Could you check a few things on this model? Use its own coordinates, in mm. Face numbers are marked on the shaded views. A direction names the side the tool comes from. Give positions to 0.01 mm unless a question says otherwise; leave off trailing zeros. Write each loop counter-clockwise with the first axis right and the second up, starting at its lowest first coordinate (ties: lowest second). Pieces come first, ordered by that corner, then holes. Notation, with made-up numbers: M 12.5,30 L 71.5,30 A21 ccw 71.5,36 Z; hole C 64,5.25 d7. An arc over 180 degrees is marked long. Answer as CSV lines item,"result". Start each with the question number.
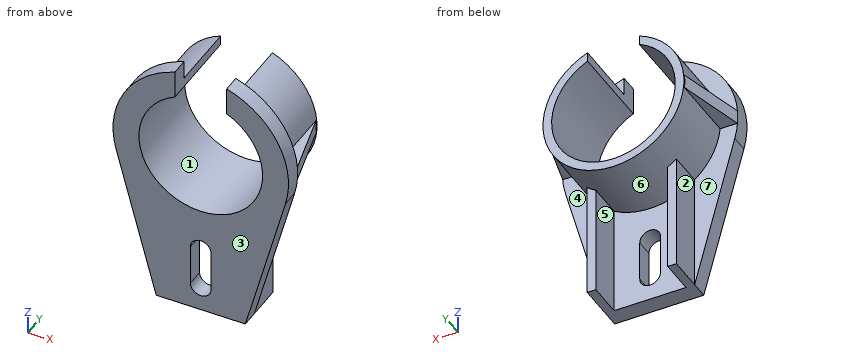
from build123d import *

# Parameters (mm, degrees)
SKETCH8_R           = 11.3665
BOSS_EXTRUDE3_DEPTH = 3.175
SKETCH9_R           = 12.954
SKETCH9_R_2         = 11.3665
BOSS_EXTRUDE4_DEPTH = 12.7
RIB12_REACH         = 40.783
SKETCH13_WALL_W     = 92.662520058
SKETCH13_WALL_H     = 2.54
CUT_EXTRUDE1_DEPTH  = 52.861115163
RIB1_START          = -47.625
RIB1_OUTLINE_W      = 1.5875
RIB1_OUTLINE_H      = 6.35
RIB1_DEPTH          = 21.4607898
SKETCH16_W          = 9.525
SKETCH16_H          = 15.588386278
CUT_EXTRUDE3_DEPTH  = 53.72855859


# Read off the part's stored shape, not the designer's step: Rib1
with BuildPart() as part:
    # Sketch8 → Boss-Extrude3 (new body)
    with BuildSketch(Plane(origin=(0, 0, 0), x_dir=(1, 0, 0), z_dir=(0, 1, 0))):
        with BuildLine():
            Line((-8.1915, 47.625), (8.1915, 47.625))
            Line((8.1915, 47.625), (15.569804863, 20.339203977))
            ThreePointArc((15.569804863, 20.339203977), (0, 0), (-15.569804863, 20.339203977))
            Line((-15.569804863, 20.339203977), (-8.1915, 47.625))
        make_face()
        with Locations(Location((0, 16.129, 0), (0, 0, 270))):
            Circle(SKETCH8_R, mode=Mode.SUBTRACT)
    extrude(amount=BOSS_EXTRUDE3_DEPTH)

    # Sketch9 → Boss-Extrude4 (add)
    with BuildSketch(Plane(origin=(0, 3.175, 0), x_dir=(1, 0, 0), z_dir=(0, 1, 0))):
        with Locations(Location((0, 16.129, 0), (0, 0, 270))):
            Circle(SKETCH9_R)
        with Locations(Location((0, 16.129, 0), (0, 0, 270))):
            Circle(SKETCH9_R_2, mode=Mode.SUBTRACT)
    extrude(amount=BOSS_EXTRUDE4_DEPTH)

    # Sketch13 wall → Rib12 (add, up to next)
    with BuildSketch(Plane(origin=(-14.453521799, 9.525, -16.129), x_dir=(-0.243924343996, -0.969794263958, 0), z_dir=(0.969794263958, -0.243924343996, 0)), mode=Mode.PRIVATE) as rib12_sk1:
        Rectangle(SKETCH13_WALL_W, SKETCH13_WALL_H)
    rib12_tool1 = extrude(rib12_sk1.sketch, amount=RIB12_REACH, mode=Mode.PRIVATE) - part.part
    rib12 = rib12_tool1.solids().sort_by_distance((-14.453521799, 9.525, -16.129))[0]
    add(rib12)

    # Mirror2: Rib12 across plane
    add(rib12.mirror(Plane(origin=(0, 0, 0), x_dir=(0, 0, 1), z_dir=(1, 0, 0))))

    # Sketch11 → Cut-Extrude1 (cut, through all)
    with BuildSketch(Plane(origin=(0, 3.175, 0), x_dir=(1, 0, 0), z_dir=(0, 1, 0))):
        with BuildLine():
            Line((1.89865, 42.8625), (1.89865, 35.433))
            ThreePointArc((1.89865, 35.433), (0, 33.53435), (-1.89865, 35.433))
            Line((-1.89865, 35.433), (-1.89865, 42.8625))
            ThreePointArc((-1.89865, 42.8625), (0, 44.76115), (1.89865, 42.8625))
        make_face()
    extrude(amount=-CUT_EXTRUDE1_DEPTH, mode=Mode.SUBTRACT)

    # Rib1 outline → Rib1 (add)
    with BuildSketch(Plane.XY.offset(RIB1_START)):
        with Locations((-7.39775, 6.35)):
            Rectangle(RIB1_OUTLINE_W, RIB1_OUTLINE_H)
    rib1 = extrude(amount=RIB1_DEPTH)

    # Mirror1: Rib1 across plane
    add(rib1.mirror(Plane(origin=(0, 0, 0), x_dir=(0, 0, 1), z_dir=(1, 0, 0))))

    # Sketch16 → Cut-Extrude3 (cut, through all)
    with BuildSketch(Plane(origin=(0, 0, 0), x_dir=(1, 0, 0), z_dir=(0, 1, 0))):
        Rectangle(SKETCH16_W, SKETCH16_H)
    extrude(amount=CUT_EXTRUDE3_DEPTH, mode=Mode.SUBTRACT)


solid = part.part
1. Imagine slicing it at C-C, the plane z = -6.5. Please give me the cut outline in (x, y) (3 decimals), plus the area to 4 significant figures.
2. On a 3-axis mill with a long thin cutter (end or side, diameter ignored), from which of +Z, -Z, +X, -X, +Y, -Y can I reach the whole of each face in a straight line? I mean the marked faces 4, 5, 6 and 7. Say none if no direction works.
3. Imagine slicing it at D-D, the plane x = -6. Please give me the cut outline in (y, z) (3 decimals).
4. Will these pins go through, and if not, where does the flat tip stop? P1, Ø14.5, axis at x = -0.5, z = -34, coming from the +Y side (3 decimals); P2, Ø4, axis at y = 8.5, z = -4.5, coming from the +X side; P3, Ø0.8, axis at x = 7.5, z = -36, coming from the +Y side (3 decimals); P4, Ø1.6, axis at y = 2, z = -39, coming from the -X side.
5. Imagine slicing it at A-A, the plane x = 0. Please give me the cut outline in (y, z) (1 decimal), plus the area to 3 significant figures.
6. Thinking about a two-plate mould opening in X: for the marked faces 1, 2 and 3, which applies, pulls with the +X half, pulls with the -X half, needs draft (parallel to the pull), parting line crosses it, or undercut?
7. Imagine slicing it at B-B, the plane y = 1.75. Please give me the cut outline in (x, z) (1 decimal).
8. Please list where these lines run through material, in increasing order: line 1 (X direction, y = 3.25, z = -44); line 2 (Z direction, x = 0, y = 12); line 3 (Y direction, x = -5.5, z = -39) (3 decimals).
Solutions:
1,outline,"M -12.939,0 L -6.04,0 L -6.04,15.875 L -8.665,15.875 L -8.665,3.175 L -12.939,3.175 Z; M 6.04,0 L 12.939,0 L 12.939,3.175 L 8.665,3.175 L 8.665,15.875 L 6.04,15.875 Z"
1,area,"110.5 mm²"
2,face 4,"+X, +Y"
2,face 5,"-Z, +Y"
2,face 6,"+Y"
2,face 7,"-X, +Y"
3,outline,"M 0,-47.625 L 3.175,-47.625 L 3.175,-27.61 L 15.875,-27.61 L 15.875,-25.783 L 0,-25.783 Z; M 0,-6.475 L 15.875,-6.475 L 15.875,-4.648 L 3.175,-4.648 L 3.175,-1.158 L 0,-1.158 Z"
4,P1,"y = 15.875"
4,P2,"x = 8.67"
4,P3,"y = 9.525"
4,P4,"x = -10.74"
5,outline,"M 0,-47.6 L 3.2,-47.6 L 3.2,-44.8 L 0,-44.8 Z; M 0,-33.5 L 3.2,-33.5 L 3.2,-29.1 L 15.9,-29.1 L 15.9,-27.5 L 0,-27.5 Z"
5,area,"48.4 mm²"
6,face 1,"undercut"
6,face 2,"pulls with the -X half"
6,face 3,"needs draft"
7,outline,"M -15.6,-20.3 L -8.2,-47.6 L 8.2,-47.6 L 15.6,-20.3 A16.1 ccw 4.8,-0.7 L 4.8,-5.8 A11.4 cw long -4.8,-5.8 L -4.8,-0.7 A16.1 ccw Z; hole M -1.9,-42.9 A1.9 ccw 1.9,-42.9 L 1.9,-35.4 A1.9 ccw -1.9,-35.4 Z"
8,line 1,"-8.19 to -6.6, 6.6 to 8.19"
8,line 2,"-29.08 to -27.5"
8,line 3,"0 to 3.175"
